Can you work these out from the model? Positions are in its coordinate system, mm. Round coordinates to 2 decimals unless told otherwise and drop trailing zeros. Loops run counter-clockwise (first coordinate to the right, second up) from the corner with the lowest first, then second, coordinate; pieces in that order, holes last.
from build123d import *

# Parameters (mm, degrees)
F0_W     = 184.15
F0_H     = 76.2
F1_DEPTH = 11.176
F2_R     = 12.7
F3_W     = 127
F3_H     = 25.4
F4_DEPTH = 11.176
F5_R     = 6.35
F7_D     = 5.1054
F8_R     = 0.8255
F10_D    = 8.7376


# Not quite as in the source:
# - a feature names something its author has since deleted; it is built from what else it names


with BuildPart() as f1:
    # F0 (on Front) → F1 (new body)
    with BuildSketch(Plane.XZ):
        Rectangle(F0_W, F0_H)
    extrude(amount=F1_DEPTH)

    # F2
    f2_edges = [f1.edges().sort_by_distance(p)[0] for p in [
        (92.075, -5.588, 38.1),
        (92.075, -5.588, -38.1),
        (-92.075, -5.588, -38.1),
        (-92.075, -5.588, 38.1),
    ]]
    fillet(f2_edges, radius=F2_R)

    # F3 (on Front) → F4 (join)
    with BuildSketch(Plane.XZ):
        with Locations((0, 50.8)):
            Rectangle(F3_W, F3_H)
        with Locations((0, -50.8)):
            Rectangle(F3_W, F3_H)
    extrude(amount=F4_DEPTH)

    # F5
    f5_edges = [f1.edges().sort_by_distance(p)[0] for p in [
        (-63.5, -5.588, 63.5),
        (-63.5, -5.588, 38.1),
        (63.5, -5.588, 63.5),
        (63.5, -5.588, 38.1),
        (-63.5, -5.588, -63.5),
        (63.5, -5.588, -63.5),
        (63.5, -5.588, -38.1),
        (-63.5, -5.588, -38.1),
    ]]
    fillet(f5_edges, radius=F5_R)

    # F7 (through all)
    with Locations(Plane(origin=(0, 0, 0), x_dir=(-1, 0, 0), z_dir=(0, 1, 0))):
        with Locations((-60.5506403027, 22.4506403027), (-15.6493596973, 22.4506403027), (-60.5506403027, -22.4506403027), (-15.6493596973, -22.4506403027), (15.6493596973, 22.4506403027), (15.6493596973, -22.4506403027), (60.5506403027, 22.4506403027), (60.5506403027, -22.4506403027)):
            Hole(F7_D / 2)

    # F8
    f8_edges = [f1.edges().sort_by_distance(p)[0] for p in [
        (0, 0, 63.5),
    ]]
    fillet(f8_edges, radius=F8_R)

    # F10 (through all)
    with Locations(Plane(origin=(0, 0, 0), x_dir=(-1, 0, 0), z_dir=(0, 1, 0))):
        with Locations((-38.1, 50.8), (0, 50.8), (-38.1, -50.8), (0, -50.8)):
            Hole(F10_D / 2)


solid = f1.part
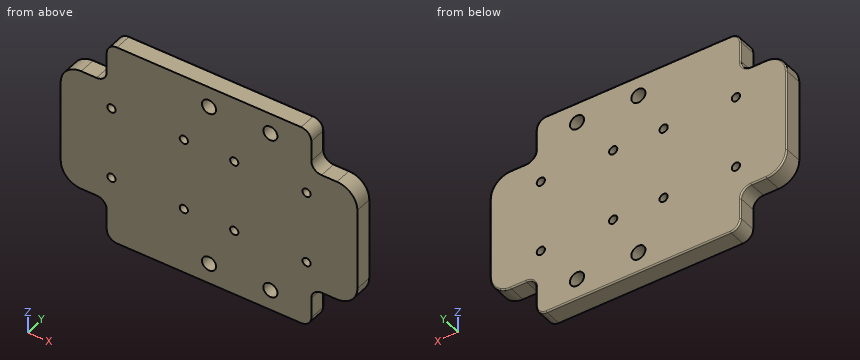
(1) If we section it at C-C, the plane y = -6.25: State how many separate pieces and enclosed holes the cut face has, then the cut area to 3 significant figures.
Worked answers:
separate pieces: 1
enclosed holes: 12
area: 19,900 mm2
(2) Will these pins go through, and if not, where does the flat tip stop? P1, Ø5, axis at y = -5, z = -34.5, coming from the -X side; P2, Ø5, axis at x = -75, y = -4, coming from the +Z side; P3, Ø5, axis at x = 74, y = -8, coming from the -Z side.
Worked answers:
P1: stops at x = -90.23
P2: stops at z = 38.1
P3: stops at z = -38.1
(3) If we section it at B-B, the plane x = 38.1: List the corners of the cut face in (y, z) for me.
Worked answers:
outline: (-11.18, -63.5) - (-0.83, -63.5) arc R0.83 ccw to (0, -62.67) - (0, -55.17) - (-11.18, -55.17) - close; (-11.18, -46.43) - (0, -46.43) - (0, 46.43) - (-11.18, 46.43) - close; (-11.18, 55.17) - (0, 55.17) - (0, 62.67) arc R0.83 ccw to (-0.83, 63.5) - (-11.18, 63.5) - close
(4) If we section it at A-A, the plane z = 50.8: List the corners of the cut face in (x, y) for me, then the cut area to 3 significant figures.
Worked answers:
outline: (-63.5, -11.18) - (-4.37, -11.18) - (-4.37, 0) - (-62.67, 0) arc R0.83 ccw to (-63.5, -0.83) - close; (4.37, -11.18) - (33.73, -11.18) - (33.73, 0) - (4.37, 0) - close; (42.47, -11.18) - (63.5, -11.18) - (63.5, -0.83) arc R0.83 ccw to (62.67, 0) - (42.47, 0) - close
area: 1,220 mm2
(5) If I drill on line 1 (Z direction, x = 0.5, y = -8); line 2 (Z direction, x = 0, y = -5.25); line 3 (X direction, y = -1, z = 23) (3 decimals), over which ranges is the centre line in solid material (lowest first)?
Worked answers:
line 1: z = -63.5 to -55.14, -46.46 to 46.46, 55.14 to 63.5
line 2: z = -63.5 to -55.17, -46.43 to 46.43, 55.17 to 63.5
line 3: x = -92.075 to -63.044, -58.058 to -18.142, -13.156 to 13.156, 18.142 to 58.058, 63.044 to 92.075
